For this review, take the finished solid that the model builds, in its own axes (mm). A direction names the side the tool comes from. Give positions to 0.01 mm unless a question says otherwise; leave off trailing zeros. Order: outer loops, then holes, each group sorted by start corner. A loop starts at its lowest first (then second) coordinate and runs counter-clockwise, first axis right, second up. Notation, with made-up numbers: M 31,-33 L 63,-33 A27 ccw 63,-5 Z; hole C 89,6.5 d7. An arc over 180 degrees is marked long. Answer as CSV lines item,"result". Start each with the question number.
1. Machinability: for faces 1 (the cylindrical face through (2.028, 224.957, -19.349)), 2 (the flat face through (20, 148, -76)), which of the approach directions +Z, -Z, +X, -X, +Y, -Y give a long, thin tool a straight path to every point of the face, cutting with its end or side? Answer none if there is none.
2. We need section D-D, the plane x = 16. Give the boundary of the cut face in (y, z).
3. Mouldability with a two-part tool opening along X and no side actions: class faces 3 (the flat face through (20, 148, -4)), 4 (the cylindrical face through (38.028, 224.957, -19.349)), 5 (the flat face through (40, 148, -39)) as pulls with the +X half, pulls with the -X half, needs draft (parallel to the pull), parting line crosses it, or undercut.
4. For line 1 along Z through (x, y) = (38.4, 260); line 2 along Y through (x, z) = (2, -60); line 3 along X through (y, z) = (154, -16.5), list the stretches that pass through material, from the lowest coordinate up.
5. We need section B-B, the plane y = 260. State how many separate pieces and enclosed holes the cut face has, and give its area (3 significant figures).
6. We need section A-A, the plane z = -71. Give the boundary of the cut face in (x, y), and give its area (3 significant figures).
7. We need section C-C, the plane z = -60. Give the boundary of the cut face in (x, y).
from build123d import *

# Parameters (mm, degrees)
BOSS_EXTRU_1_DEPTH      = 300
ESQUISSE3_R             = 12.5
ENL_V_MAT_EXTRU_1_DEPTH = 314.04951685
ESQUISSE4_R             = 5
ENL_V_MAT_EXTRU_2_DEPTH = 314.04951685


with BuildPart() as part:
    # Esquisse2 → Boss.-Extru.1 (new body)
    with BuildSketch(Plane(origin=(0, 0, 0), x_dir=(1, 0, 0), z_dir=(0, 1, 0))):
        with BuildLine():
            Line((2, 0), (38, 0))
            ThreePointArc((38, 0), (39.414213562, 0.585786438), (40, 2))
            Line((40, 2), (40, 78))
            ThreePointArc((40, 78), (39.414213562, 79.414213562), (38, 80))
            Line((38, 80), (2, 80))
            ThreePointArc((2, 80), (0.585786438, 79.414213562), (0, 78))
            Line((0, 78), (0, 2))
            ThreePointArc((0, 2), (0.585786438, 0.585786438), (2, 0))
        make_face()
        with BuildLine():
            Line((6, 4), (34, 4))
            ThreePointArc((34, 4), (35.414213562, 4.585786438), (36, 6))
            Line((36, 6), (36, 74))
            ThreePointArc((36, 74), (35.414213562, 75.414213562), (34, 76))
            Line((34, 76), (6, 76))
            ThreePointArc((6, 76), (4.585786438, 75.414213562), (4, 74))
            Line((4, 74), (4, 6))
            ThreePointArc((4, 6), (4.585786438, 4.585786438), (6, 4))
        make_face(mode=Mode.SUBTRACT)
    extrude(amount=BOSS_EXTRU_1_DEPTH)

    # Esquisse3 → Enlèv. mat.-Extru.1 (cut, through all)
    with BuildSketch(Plane(origin=(40, 0, 0), x_dir=(0, 0, -1), z_dir=(1, 0, 0))):
        with Locations((40, 40)):
            Circle(ESQUISSE3_R)
    extrude(amount=-ENL_V_MAT_EXTRU_1_DEPTH, mode=Mode.SUBTRACT)

    # Esquisse4 → Enlèv. mat.-Extru.2 (cut, through all)
    with BuildSketch(Plane(origin=(40, 0, 0), x_dir=(0, 0, -1), z_dir=(1, 0, 0))):
        with Locations((60, 220)):
            Circle(ESQUISSE4_R)
        with Locations((20, 220)):
            Circle(ESQUISSE4_R)
        with Locations((20, 260)):
            Circle(ESQUISSE4_R)
        with Locations((60, 260)):
            Circle(ESQUISSE4_R)
    extrude(amount=-ENL_V_MAT_EXTRU_2_DEPTH, mode=Mode.SUBTRACT)


solid = part.part
Result set:
1,face 1,"+X, -X"
1,face 2,"+Y, -Y"
2,outline,"M 0,-80 L 300,-80 L 300,-76 L 0,-76 Z; M 0,-4 L 300,-4 L 300,0 L 0,0 Z"
3,face 3,"undercut"
3,face 4,"needs draft"
3,face 5,"pulls with the +X half"
4,line 1,"-79.96 to -65, -55 to -25, -15 to -0.04"
4,line 2,"0 to 215, 225 to 255, 265 to 300"
4,line 3,"0 to 4, 36 to 40"
5,separate pieces,"4"
5,enclosed holes,"0"
5,area,"736 mm2"
6,outline,"M 0,0 L 4,0 L 4,300 L 0,300 Z; M 36,0 L 40,0 L 40,300 L 36,300 Z"
6,area,"2,400 mm2"
7,outline,"M 0,0 L 4,0 L 4,215 L 0,215 Z; M 0,225 L 4,225 L 4,255 L 0,255 Z; M 0,265 L 4,265 L 4,300 L 0,300 Z; M 36,0 L 40,0 L 40,215 L 36,215 Z; M 36,225 L 40,225 L 40,255 L 36,255 Z; M 36,265 L 40,265 L 40,300 L 36,300 Z"
